```python
from build123d import *

# Parameters (mm, degrees)
EXTRUDE_1_DEPTH     = 5
SKETCH_8_OUTSIDE_W  = 22.464
SKETCH_8_OUTSIDE_H  = 20.522
SKETCH_8_OUTSIDE_R  = 6.278684177
CUT_EXTRUDE_1_DEPTH = 1
CUT_EXTRUDE_1_TAPER = 45
SKETCH_9_R          = 3.825
BOLT_LENGTH_DEPTH   = 55
FILLET_1_R          = 1
CHAMFER_1_SIZE      = 1


with BuildPart() as part:
    # Эскиз6 → Бобышка-Вытянуть1 (new body)
    with BuildSketch(Plane(origin=(0, 0, 0), x_dir=(1, 0, 0), z_dir=(0, 1, 0))):
        Polygon((7.25, 0), (3.625, 6.278684177), (-3.625, 6.278684177), (-7.25, 0), (-3.625, -6.278684177), (3.625, -6.278684177), align=None)
    extrude(amount=EXTRUDE_1_DEPTH)

    # Эскиз8 outside → Вырез-Вытянуть1 (cut)
    with BuildSketch(Plane(origin=(0, 5, 0), x_dir=(1, 0, 0), z_dir=(0, 1, 0))):
        Rectangle(SKETCH_8_OUTSIDE_W, SKETCH_8_OUTSIDE_H)
        Circle(SKETCH_8_OUTSIDE_R, mode=Mode.SUBTRACT)
    extrude(amount=-CUT_EXTRUDE_1_DEPTH, taper=CUT_EXTRUDE_1_TAPER, mode=Mode.SUBTRACT)

    # Эскиз9 → bolt length (add)
    with BuildSketch(Plane.XZ):
        Circle(SKETCH_9_R)
    extrude(amount=BOLT_LENGTH_DEPTH)

    # Скругление1
    fillet_1_edges = [part.edges().sort_by_distance(p)[0] for p in [
        (-3.825, 0, 0),
    ]]
    fillet(fillet_1_edges, radius=FILLET_1_R)

    # Фаска1
    chamfer_1_edges = [part.edges().sort_by_distance(p)[0] for p in [
        (-3.825, -55, 0),
    ]]
    chamfer(chamfer_1_edges, length=CHAMFER_1_SIZE)


solid = part.part
```
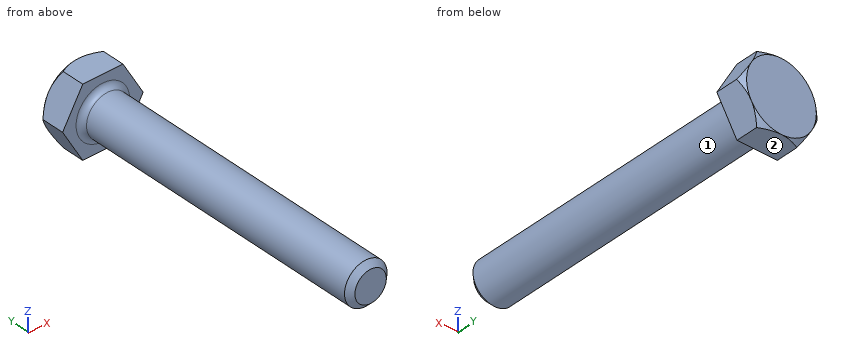
Work out the finished part from the listing and answer in its coordinate system (mm). Face numbers are marked on the shaded views. A direction names the side the tool comes from. Give positions to 0.01 mm unless a question says otherwise; leave off trailing zeros. Order: outer loops, then holes, each group sorted by start corner. A loop starts at its lowest first (then second) coordinate and runs counter-clockwise, first axis right, second up. Notation, with made-up numbers: (20.25, 89) - (67.25, 89) arc R22 cw to (67.25, 95) - close; hole circle Ø6 at (-22.5, 26.25). An arc over 180 degrees is marked (long way). One line per item, written item: value. Start each with the question number.
1. Which of the six approach directions +Z, -Z, +X, -X, +Y, -Y give full straight-line access (tool end or side, diameter ignored) to the marked faces 1 and 2?
2. This flat-tipped pin is pushed along its axis until it touches: pin 1 Ø3 at (x, y) = (-1.5, -14.5) entering from -Z (3 decimals). Where does it stop, or does it pass through?
3. Consider line 1 (Y direction, x = 0, z = 5.25); line 2 (X direction, y = -15.5, z = -0.25); line 3 (Z direction, x = 2.25, y = -14). Determine where each line is inside the solid, lowest interval first.
4. Section A-A, the plane y = -16 is taken. Write down the section's boundary in (x, z) (3 decimals).
Filled sheet:
1. face 1: -Y
1. face 2: -Z, +X, -X, +Y, -Y
2. pin 1: z = -3.825
3. line 1: 0 to 5
3. line 2: -3.82 to 3.82
3. line 3: -3.09 to 3.09
4. outline: circle Ø7.65 at (0, 0)
